The model under review builds one solid part; all positions refer to its coordinate system, in mm. A direction names the side the tool comes from. Coordinates: 2 decimals unless noted, no trailing zeros. Write each loop counter-clockwise with the first axis right and the second up, starting at its lowest first coordinate (ties: lowest second). Pieces come first, ordered by that corner, then holes. Notation, with made-up numbers: M 35,7 L 39,7 A12 cw 39,16 Z; hole C -4.5,19 d1. An arc over 180 degrees is marked long. Answer as a JSON object with one key per item and string values.
```python
from build123d import *

# Parameters (mm, degrees)
F1_DEPTH = 12.7
F4_DEPTH = 6.35
F5_R     = 3.175
F6_DEPTH = 76.201


# Not quite as in the source:
# - a feature of the source that left no trace in its solid (it failed there, or was rolled back) is left out


with BuildPart() as f1:
    # F0 (on Front) → F1 (new body, symmetric)
    with BuildSketch(Plane.XZ):
        Polygon((0, 38.1), (0, 0), (76.2, 0), (76.2, 12.7), (50.8, 12.7), (50.8, 38.1), (38.1, 38.1), (38.1, 50.8), (12.7, 50.8), align=None)
    extrude(amount=F1_DEPTH, both=True)

    # F2 (on Front) → F4 (cut, symmetric)
    with BuildSketch(Plane.XZ):
        Polygon((38.1, 50.8), (25.4, 50.8), (25.4, 25.4), (50.8, 25.4), (50.8, 38.1), (38.1, 38.1), align=None)
    extrude(amount=F4_DEPTH, both=True, mode=Mode.SUBTRACT)

    # F5 (on Right) → F6 (cut, through all)
    with BuildSketch(Plane.YZ):
        with Locations((0, 12.7)):
            Circle(F5_R)
    extrude(amount=F6_DEPTH, mode=Mode.SUBTRACT)


solid = f1.part
```
(1) Add section D-D on y = 4. Give the boundary of the cut face in (x, z).
Results list:
{"outline": "M 0,0 L 76.2,0 L 76.2,12.7 L 50.8,12.7 L 50.8,25.4 L 25.4,25.4 L 25.4,50.8 L 12.7,50.8 L 0,38.1 Z"}
(2) Wall thickness on line 1 along Z through (x, y) = (41, 0) (3 decimals); line 2 along Y through (x, z) = (30, 12.7) (3 decimals); line 3 along Y through (x, z) = (35.5, 26.5): over which ranges is each line inside the solid? List them lowest first. Write a range as from..to.
Results list:
{"line 1": "0..9.525, 15.875..25.4", "line 2": "-12.7..-3.175, 3.175..12.7", "line 3": "-12.7..-6.35, 6.35..12.7"}
(3) For faces 4 (the face through (35, 6.35, 35)), 5 (the face through (29, 12.7, 20)), 6 (the face through (38.1, 9, 44)), list the 3-axis set-ups (+Z, -Z, +X, -X, +Y, -Y) from which the entire face can be reached by the end or side of a thin tool; tool diameter is ignored.
Results list:
{"face 4": "+Z, +X", "face 5": "+Z, -Z, +X, -X, +Y", "face 6": "+Z, +X, +Y, -Y"}
(4) Add section B-B on x = 5. Give the boundary of the cut face in (y, z) (3 decimals), and give its area (3 significant figures).
Results list:
{"outline": "M -12.7,0 L 12.7,0 L 12.7,43.1 L -12.7,43.1 Z; hole C 0,12.7 d6.35", "area": "1,060 mm²"}
(5) Draft analysis for pull direction Z (two halves, no side actions). For faces 1 (the face through (38, 0, 0)), 2 (the face through (29.1, 1.5, 9.9)), 3 (the face through (35, -6.35, 35)), state which applies: released by +Z, released by -Z, zero draft, split by the parting line, or undercut.
Results list:
{"face 1": "released by -Z", "face 2": "undercut", "face 3": "zero draft"}
(6) For pin 1 Ø7 at (y, z) = (-11, 44.5) entering from +X; pin 2 Ø5 at (x, y) = (63.5, 10) entering from +Z; pin 3 Ø7.5 at (y, z) = (-2.5, 21.5) entering from +X, all flat-tipped, find the tip position at first contact; note any pin that passes through.
Results list:
{"pin 1": "x = 38.1", "pin 2": "z = 12.7", "pin 3": "x = 50.8"}
(7) Add section C-C on z = 33.5. Give the boundary of the cut face in (x, y), and give its area (3 significant figures).
Results list:
{"outline": "M 0,-12.7 L 50.8,-12.7 L 50.8,-6.35 L 25.4,-6.35 L 25.4,6.35 L 50.8,6.35 L 50.8,12.7 L 0,12.7 Z", "area": "968 mm²"}
(8) Add section A-A on y = 0. Give the boundary of the cut face in (x, z) (3 decimals), and give its area (3 significant figures).
Results list:
{"outline": "M 0,0 L 76.2,0 L 76.2,9.525 L 0,9.525 Z; M 0,15.875 L 50.8,15.875 L 50.8,25.4 L 25.4,25.4 L 25.4,50.8 L 12.7,50.8 L 0,38.1 Z", "area": "1,770 mm²"}
